```python
from build123d import *

# Parameters (mm, degrees)
SKETCH1_R           = 10.668
SKETCH1_R_2         = 7.8994
BOSS_EXTRUDE1_DEPTH = 50.8
SKETCH2_R           = 10.668
SKETCH2_R_2         = 7.8994
BOSS_EXTRUDE2_DEPTH = 33.02
SKETCH3_R           = 7.8994
CUT_EXTRUDE1_DEPTH  = 51.8000001
CUT_EXTRUDE2_REACH  = 45.688
SKETCH4_R           = 7.8994


with BuildPart() as part:
    # Sketch1 → Boss-Extrude1 (new body)
    with BuildSketch(Plane.XY):
        Circle(SKETCH1_R)
        Circle(SKETCH1_R_2, mode=Mode.SUBTRACT)
    extrude(amount=BOSS_EXTRUDE1_DEPTH)

    # Sketch2 → Boss-Extrude2 (add)
    with BuildSketch(Plane(origin=(0, 0, 0), x_dir=(1, 0, 0), z_dir=(0, 1, 0))):
        with Locations((0, -25.4)):
            Circle(SKETCH2_R)
        with Locations((0, -25.4)):
            Circle(SKETCH2_R_2, mode=Mode.SUBTRACT)
    extrude(amount=BOSS_EXTRUDE2_DEPTH)

    # Sketch3 → Cut-Extrude1 (cut, through all)
    with BuildSketch(Plane.XY.offset(50.8)):
        Circle(SKETCH3_R)
    extrude(amount=-CUT_EXTRUDE1_DEPTH, mode=Mode.SUBTRACT)

    # Sketch4 → Cut-Extrude2 (cut, up to next)
    with BuildSketch(Plane(origin=(0, 33.02, 0), x_dir=(1, 0, 0), z_dir=(0, 1, 0)), mode=Mode.PRIVATE) as cut_extrude2_sk1:
        with Locations((0, -25.4)):
            Circle(SKETCH4_R)
    cut_extrude2_tool1 = extrude(cut_extrude2_sk1.sketch, amount=-CUT_EXTRUDE2_REACH, mode=Mode.PRIVATE) & part.part
    add(cut_extrude2_tool1.solids().sort_by_distance((0, 33.02, 25.4))[0], mode=Mode.SUBTRACT)


solid = part.part
```
Input: part model. Units: mm. Frame: model coordinates. A direction names the side the tool comes from. Coordinates: 2 decimals unless noted, no trailing zeros. Loops run counter-clockwise (first coordinate to the right, second up) from the corner with the lowest first, then second, coordinate; pieces in that order, holes last. Notation, with made-up numbers: M 24.5,-18 L 63.5,-18 A34 ccw 63.5,15 Z; hole C 27,-20.5 d3. An arc over 180 degrees is marked long. Use a Markdown table: item, result. Add a question column.
1) Line query: L1, parallel to Z at x = 0, y = 24.75; L2, parallel to X at y = 5, z = 25; L3, parallel to Z at x = 0, y = 8.5. Output: solid intervals per line, ascending. Write a range as from..to.
2) Section B-B, the plane z = 25.4. Return the cut outline in (x, y), plus the area to 3 significant figures.
3) Section D-D, the plane y = 16.5. Return the cut outline in (x, z).
4) Set-up query: faces 4 (the cylindrical face through (-10.658, 19.948, 24.931)), 5 (the flat face through (-7, -4, 0)). Return all of +Z, -Z, +X, -X, +Y, -Y with unobstructed straight access to the full face (end or side cutting, diameter ignored); none if empty.
5) Section C-C, the plane y = 1.5. Return the cut outline in (x, z), plus the area to 3 significant figures.
6) Draft query along Y for faces 1 (the cylindrical face through (4.923, -9.464, 25.044)), 2 (the flat face through (0, 33.02, 17)), 3 (the cylindrical face through (-1.712, -7.712, 25.044)). Return one class per face: +Y half, -Y half, draft (parallel to the pull), parting line (faces both ways), or undercut.
7) Pin query (flat end, axial travel): P1, Ø2, axis at x = 5, z = 15, coming from the -Y side; P2, Ø9.5, axis at x = 0, z = 25.4, coming from the +Y side; P3, Ø9.5, axis at x = 0, y = 0, coming from the +Z side; P4, Ø5, axis at x = -1, z = 9.5, coming from the -Y side. Return the tip coordinate at first contact, or that it passes through.
8) Section A-A, the plane x = 0. Return the cut outline in (y, z).
Answer below:
| question | item | result |
|---|---|---|
| 1 | L1 | 14.73..17.5, 33.3..36.07 |
| 1 | L2 | -10.66..-7.89, 7.89..10.66 |
| 1 | L3 | 0..17.5, 33.3..50.8 |
| 2 | outline | M -10.67,0 A10.67 ccw 10.67,0 L 10.67,33.02 L 7.9,33.02 L 7.9,0 A7.9 cw -7.9,0 L -7.9,33.02 L -10.67,33.02 Z |
| 2 | area | 264 mm2 |
| 3 | outline | C 0,25.4 d21.34; hole C 0,25.4 d15.8 |
| 4 | face 4 | +Y |
| 4 | face 5 | -Z, +X, -X, +Y, -Y |
| 5 | outline | M -10.56,0 L -7.76,0 L -7.76,23.9 A7.9 cw -7.76,26.9 L -7.76,50.8 L -10.56,50.8 L -10.56,26.9 A10.67 ccw -10.56,23.9 Z; M 7.76,0 L 10.56,0 L 10.56,23.9 A10.67 ccw 10.56,26.9 L 10.56,50.8 L 7.76,50.8 L 7.76,26.9 A7.9 cw 7.76,23.9 Z |
| 5 | area | 285 mm2 |
| 6 | face 1 | parting line |
| 6 | face 2 | +Y half |
| 6 | face 3 | undercut |
| 7 | P1 | y = -9.89 |
| 7 | P2 | y = -6.31 |
| 7 | P3 | through |
| 7 | P4 | y = -10.67 |
| 8 | outline | M -10.67,0 L -7.9,0 L -7.9,50.8 L -10.67,50.8 Z; M 7.9,0 L 10.67,0 L 10.67,14.73 L 33.02,14.73 L 33.02,17.5 L 7.9,17.5 Z; M 7.9,33.3 L 33.02,33.3 L 33.02,36.07 L 10.67,36.07 L 10.67,50.8 L 7.9,50.8 Z |
